Model file for the job. Use its own axes, mm. Face numbers are marked on the shaded views. A direction names the side the tool comes from. Round coordinates to 2 decimals unless told otherwise and drop trailing zeros. Loops run counter-clockwise (first coordinate to the right, second up) from the corner with the lowest first, then second, coordinate; pieces in that order, holes last. Notation, with made-up numbers: (-22, -25.5) -> (11, -25.5) arc R15 cw to (11, -1.5) -> close; hole circle Ø2 at (47, 49). An arc over 180 degrees is marked (long way). Use a Markdown table: item, result. Add a question column.
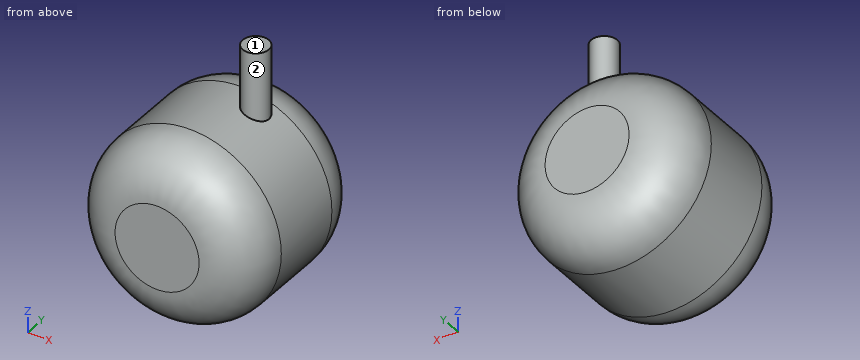
```python
from build123d import *

# Parameters (mm, degrees)
F0_R     = 19.8247
F1_DEPTH = 38.1
F2_R     = 10.731179
F3_R     = 2.8448
F4_DEPTH = 49.53


with BuildPart() as f1:
    # F0 (on Front) → F1 (new body)
    with BuildSketch(Plane.XZ):
        with Locations((-19.473333, 16.51)):
            Circle(F0_R)
    extrude(amount=F1_DEPTH)

    # F2
    f2_edges = [f1.edges().sort_by_distance(p)[0] for p in [
        (-39.298033, -38.1, 16.51),
        (-39.298033, 0, 16.51),
    ]]
    fillet(f2_edges, radius=F2_R)

    # F3 (on Top) → F4 (join)
    with BuildSketch(Plane.XY):
        with Locations((-13.739159, -14.360067)):
            Circle(F3_R)
    extrude(amount=F4_DEPTH)


solid = f1.part
```
1) Pin check, flat tips, straight feed: pin 1 Ø5 at (x, z) = (-23.5, 37) entering from +Y; pin 2 Ø10 at (x, y) = (-13, -30) entering from +Z; pin 3 Ø1 at (x, y) = (-12.5, -8) entering from -Z. Stop position of each tip, or through.
2) Wall check: probe 1 along Z at (x, y) = (-17, -2); probe 2 along X at (y, z) = (-12, 40); probe 3 along Z at (x, y) = (-2, -26.5). Give the ranges that are in metal, low to high. Write a range as from..to.
3) Cut at A-A on y = -20. Write the cut outline in (x, z), and give its area (3 significant figures).
4) Tool access for the marked faces 1 and 2: list every direction of +Z, -Z, +X, -X, +Y, -Y with a clear straight run to the whole face (end or side of a thin tool).
Established:
| question | item | result |
|---|---|---|
| 1 | pin 1 | stops at y = -5.36 |
| 1 | pin 2 | stops at z = 36.23 |
| 1 | pin 3 | stops at z = -1.9 |
| 2 | probe 1 | z = 1.38..31.64 |
| 2 | probe 2 | x = -15.33..-12.15 |
| 2 | probe 3 | z = 7.15..25.87 |
| 3 | outline | circle Ø39.65 at (-19.47, 16.51) |
| 3 | area | 1,230 mm^2 |
| 4 | face 1 | +Z, +X, -X, +Y, -Y |
| 4 | face 2 | +Z |
